Input: part model. Units: mm. Frame: model coordinates. Face numbers are marked on the shaded views. A direction names the side the tool comes from. Give positions to 0.01 mm unless a question says otherwise; leave off trailing zeros. Loops run counter-clockwise (first coordinate to the right, second up) from the corner with the lowest first, then second, coordinate; pieces in that order, holes last. Notation, with made-up numbers: (9.5, 78.25) - (66.5, 78.25) arc R32 cw to (66.5, 112.25) - close; hole circle Ø3 at (-13, 9.25). An arc over 180 degrees is marked (long way). Answer as a JSON object with one key per item and string values.
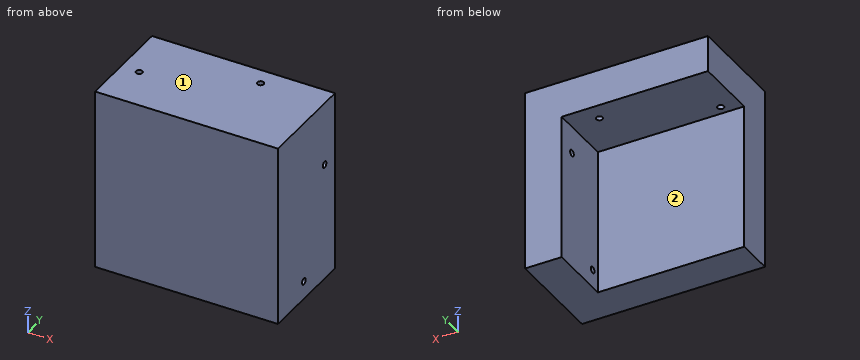
Autodesk Inventor part; units mm, degrees
ref_plane "YZ Plane" through (0, 0, 0) normal (1, 0, 0) x (0, 1, 0)
ref_plane "XZ Plane" through (0, 0, 0) normal (0, 1, 0) x (-1, 0, 0)
ref_plane "XY Plane" through (0, 0, 0) normal (0, 0, 1) x (1, 0, 0)
sketch "Boceto2" plane through (0, 0, 0) normal (0, 1, 0) x (-1, 0, 0)
  line L0 (7.5, 100) -> (-7.5, 100)
  line L1 (-7.5, 100) -> (-7.5, -100)
  line L2 (-7.5, -100) -> (7.5, -100)
  line L3 (7.5, -100) -> (7.5, 100)
  line L4 (7.5, 100) -> (-7.5, -100) construction
  line L5 (-7.5, 100) -> (7.5, -100) construction
  point P0 (0, 0)
  dimension "d7" = 15
  dimension "d8" = 200
extrude "Extrusión1" add sketch "Boceto2" along normal blind 10
sketch "Boceto3" plane through (0, 10, 0) normal (0, 1, 0) x (1, 0, 0)
  circle A0 centre (3.25, 58.25) radius 1.75
  line L0 (5, 50) -> (-5, 50)
  line L1 (-5, 50) -> (-5, 60)
  line L2 (-5, 60) -> (5, 60)
  line L3 (5, 60) -> (5, 50)
  line L4 (5, 50) -> (-5, 60) construction
  line L5 (-5, 50) -> (5, 60) construction
  circle A1 centre (-3.25, 51.75) radius 1.75
  line L6 (7.5, 100) -> (-7.5, 100)
  line L7 (-7.5, 0) -> (3.408, 0)
  line L8 (5, -60) -> (5, -50)
  line L9 (-5, -60) -> (5, -60)
  line L10 (5, -50) -> (-5, -50)
  line L11 (-5, -50) -> (-5, -60)
  line L12 (-5, -50) -> (5, -60) construction
  circle A2 centre (-3.25, -51.75) radius 1.75
  line L13 (5, -50) -> (-5, -60) construction
  circle A3 centre (3.25, -58.25) radius 1.75
  line L14 (-7.5, -100) -> (7.5, -100)
  point P0 (0, 0)
  point P1 (-5, 55)
  point P2 (0, 100)
  point P3 (-5, -55)
  dimension "d11" = 3.5
  dimension "d12" = 1.75
  dimension "d13" = 1.75
  dimension "d14" = 1.75
  dimension "d15" = 1.75
  dimension "d16" = 10
  dimension "d17" = 10
  dimension "d19" = 40
  dimension "d81" = 40
hole "Agujero1" at (3.25, 10, 58.25) at (-3.25, 10, 51.75) at (3.25, 10, -58.25) at (-3.25, 10, -51.75) direction (0, -1, 0) diameter 3.5 end through all
sketch "Boceto4" plane through (0, 10, 0) normal (0, 1, 0) x (1, 0, 0)
  line L0 (-7.5, 100) -> (-7.5, -100)
  line L1 (-7.5, -100) -> (7.5, -100)
  line L2 (7.5, -100) -> (7.5, -80)
  line L3 (7.5, -80) -> (-7.5, -80)
  line L4 (-7.5, -80) -> (-7.5, -100)
  line L5 (-7.5, 0) -> (1.0116, 0)
  line L6 (-7.5, -100) -> (-7.5, 100)
  line L7 (-7.5, 100) -> (7.5, 100)
  line L8 (7.5, 100) -> (7.5, 80)
  line L9 (7.5, 80) -> (-7.5, 80)
  line L10 (-7.5, 80) -> (-7.5, 100)
  point P0 (0, 0)
  point P1 (-7.5, -80)
  point P2 (-7.5, 80)
  dimension "d27" = 15
  dimension "d28" = 20
extrude "Extrusión2" add sketch "Boceto4" along normal blind 80
sketch "Boceto5" plane through (0, 90, 0) normal (0, 1, 0) x (1, 0, 0)
  line L0 (-7.5, -100) -> (7.5, -100)
  line L1 (-7.5, -100) -> (49.5, -100)
  line L2 (49.5, -100) -> (49.5, 100)
  line L3 (49.5, 100) -> (-7.5, 100)
  line L4 (-7.5, 100) -> (-7.5, -100)
  line L5 (49.5, -100) -> (-150.5, -100)
  line L6 (-150.5, -100) -> (-150.5, 100)
  line L7 (-150.5, 100) -> (49.5, 100)
  line L8 (49.5, 100) -> (49.5, -100)
  point P0 (0, 0)
  point P1 (-7.5, 100)
  dimension "d31" = 57
  dimension "d32" = 200
  dimension "d75" = 200
extrude "Extrusión3" add sketch "Boceto5" along normal blind 110
sketch "Boceto6" plane through (0, 200, 0) normal (0, 1, 0) x (1, 0, 0)
  line L0 (49.5, 100) -> (7.5, 100)
  line L1 (49.5, 100) -> (29.5, 100)
  line L2 (29.5, 100) -> (29.5, 80)
  line L3 (7.5, -100) -> (49.5, -100)
  line L4 (28.5, -100) -> (28.5, -80)
  line L5 (-150.5, 100) -> (-150.5, -100)
  line L6 (29.5, 80) -> (-150.5, 80)
  line L7 (-150.5, 80) -> (-150.5, -80)
  line L8 (-150.5, -80) -> (29.5, -80)
  line L9 (29.5, -80) -> (29.5, 80)
  line L10 (-150.5, -100) -> (49.5, -100)
  point P0 (7.5, 80)
  point P1 (-50.5, -100)
  dimension "d36" = 20
  dimension "d37" = 20
  dimension "d38" = 20
  dimension "d77" = 20
extrude "Extrusión4" cut sketch "Boceto6" against normal blind 90 contours L8 L5 L6 L9
sketch "Boceto7" plane through (-150.5, 90, -100) normal (-1, 0, 0) x (0, 0, 1)
  line L0 (0, 110) -> (20, 110)
  line L1 (20, 110) -> (10, 110)
  line L2 (10, 110) -> (10, 20)
  line L3 (10, 20) -> (20, 20)
  line L4 (20, 20) -> (20, 110)
  line L5 (180, 110) -> (180, 20)
  line L6 (180, 110) -> (190, 110)
  line L7 (190, 110) -> (190, 20)
  line L8 (190, 20) -> (180, 20)
  line L9 (180, 20) -> (180, 110)
  line L10 (200, 0) -> (200, 110)
  line L11 (0, 0) -> (0, 110)
  line L12 (0, 110) -> (10, 110)
  line L13 (10, 110) -> (10, 20)
  line L14 (10, 20) -> (0, 20)
  line L15 (0, 20) -> (0, 110)
  line L16 (200, 110) -> (0, 110)
  line L17 (200, 110) -> (190, 110)
  line L18 (190, 110) -> (190, 20)
  line L19 (190, 20) -> (200, 20)
  line L20 (200, 20) -> (200, 110)
  point P0 (100, -90)
  dimension "d63" = 10
  dimension "d65" = 10
  dimension "d76" = 10
extrude "Extrusión5" cut sketch "Boceto7" against normal blind 30 contours L6 L7 L8 L5 | L0 L4 L3 L2
sketch "Boceto8" plane through (-7.5, 0, 100) normal (0, 0, 1) x (1, 0, 0)
  line L0 (-113, 110) -> (-113, 200)
  line L1 (-113, 200) -> (-113, 110)
  circle A0 centre (-124.75, 183.25) radius 1.75
  line L2 (-123, 175) -> (-133, 175)
  line L3 (-133, 175) -> (-133, 185)
  line L4 (-133, 185) -> (-123, 185)
  line L5 (-123, 185) -> (-123, 175)
  line L6 (-123, 175) -> (-133, 185) construction
  line L7 (-133, 175) -> (-123, 185) construction
  circle A1 centre (-131.25, 176.75) radius 1.75
  line L8 (-143, 200) -> (57, 200)
  line L9 (-143, 90) -> (-143, 200)
  line L10 (-113, 155) -> (-128, 155)
  line L11 (-123, 125) -> (-123, 135)
  line L12 (-133, 125) -> (-123, 125)
  line L13 (-123, 135) -> (-133, 125) construction
  line L14 (-123, 135) -> (-133, 135)
  line L15 (-133, 135) -> (-123, 125) construction
  circle A2 centre (-131.25, 133.25) radius 1.75
  line L16 (-133, 135) -> (-133, 125)
  circle A3 centre (-124.75, 126.75) radius 1.75
  line L17 (-143, 110) -> (-113, 110)
  point P0 (7.5, 0)
  point P1 (-133, 180)
  point P2 (-123, 180)
  point P3 (-133, 130)
  point P4 (-123, 130)
  dimension "d45" = 3.5
  dimension "d46" = 1.75
  dimension "d47" = 1.75
  dimension "d48" = 1.75
  dimension "d49" = 1.75
  dimension "d50" = 10
  dimension "d51" = 10
  dimension "d52" = 15
  dimension "d53" = 10
  dimension "d54" = 10
  dimension "d55" = 15
hole "Agujero2" at (-132.25, 183.25, 100) at (-138.75, 176.75, 100) at (-138.75, 133.25, 100) at (-132.25, 126.75, 100) direction (0, 0, -1) diameter 3.5 end through all
ref_plane "Plano de trabajo1" through (-150.5, 90, 100) normal (0, -1, 0) x (1, 0, 0)
split "Dividir1" plane through (-150.5, 90, 100) removes the side toward (0, -1, 0)
ref_plane "Plano de trabajo2" through (49.5, 90, 0) normal (0, 0, -1) x (-1, 0, 0)
ref_plane "Plano de trabajo3" through (-50.5, 90, 100) normal (1, 0, 0) x (0, 0, -1)
ref_plane "Plano de trabajo4" through (0, 145, 0) normal (0, 1, 0) x (1, 0, 0)
sketch "Boceto9" plane through (-150.5, 90, 100) normal (0, 0, 1) x (1, 0, 0)
  line L0 (85.0357, 30) -> (115.0357, 30)
  circle A0 centre (110.0357, 25) radius 1.75
  line L1 (90.0357, 25) -> (110.0357, 25)
  line L2 (115.0357, 30) -> (115.0357, 20)
  circle A1 centre (90.0357, 25) radius 1.75
  line L3 (85.0357, 20) -> (115.0357, 30) construction
  line L4 (85.0357, 30) -> (115.0357, 20) construction
  line L5 (85.0357, 20) -> (85.0357, 30)
  line L6 (115.0357, 20) -> (85.0357, 20)
  line L7 (200, 0) -> (200, 110)
  line L8 (200, 55) -> (88.2857, 55)
  circle A2 centre (90.0357, 85) radius 1.75
  line L9 (85.0357, 80) -> (115.0357, 80)
  line L10 (85.0357, 80) -> (115.0357, 90) construction
  line L11 (85.0357, 90) -> (85.0357, 80)
  line L12 (115.0357, 90) -> (85.0357, 90)
  line L13 (85.0357, 90) -> (115.0357, 80) construction
  circle A3 centre (110.0357, 85) radius 1.75
  line L14 (90.0357, 85) -> (110.0357, 85)
  line L15 (115.0357, 80) -> (115.0357, 90)
  line L16 (100.0357, 55) -> (185.099, 55) construction
  line L17 (160, 70) -> (160, 40)
  circle A4 centre (165, 45) radius 1.75
  line L18 (170, 40) -> (170, 70)
  line L19 (170, 70) -> (160, 40) construction
  line L20 (160, 40) -> (170, 40)
  line L21 (160, 70) -> (170, 40) construction
  circle A5 centre (165, 65) radius 1.75
  line L22 (165, 65) -> (165, 45)
  line L23 (170, 70) -> (160, 70)
  circle A6 centre (55, 65) radius 1.75
  line L24 (60, 70) -> (60, 40)
  line L25 (60, 40) -> (50, 40)
  circle A7 centre (55, 45) radius 1.75
  line L26 (55, 65) -> (55, 45)
  line L27 (60, 70) -> (50, 40) construction
  line L28 (50, 40) -> (50, 70)
  line L29 (50, 70) -> (60, 40) construction
  line L30 (50, 70) -> (60, 70)
  line L31 (30, 110) -> (30, 20)
  point P0 (150.5, -90)
  point P1 (100.0357, 34.7141)
  point P2 (100.0357, 34.7141)
  point P3 (85.0357, 36.6749)
  point P4 (115.0357, 25)
  point P5 (115.0357, 85)
  point P6 (189.1833, 40)
  point P7 (165, 70)
  point P8 (70.0357, 40)
  point P9 (55, 70)
  dimension "d89" = 10
  dimension "d90" = 30
  dimension "d91" = 5
  dimension "d92" = 5
  dimension "d93" = 5
  dimension "d94" = 5
  dimension "d95" = 30
  dimension "d96" = 5
  dimension "d97" = 5
  dimension "d98" = 3.5
  dimension "d99" = 5
  dimension "d100" = 5
  dimension "d101" = 5
  dimension "d102" = 5
  dimension "d103" = 5
  dimension "d104" = 20
hole "Agujero3" at (-60.4643, 175, 100) at (-40.4643, 175, 100) at (14.5, 155, 100) at (-95.5, 155, 100) at (-95.5, 135, 100) at (-60.4643, 115, 100) at (-40.4643, 115, 100) at (14.5, 135, 100) direction (0, 0, -1) diameter 3.5 end through all
sketch "Boceto10" plane through (49.5, 90, 100) normal (1, 0, 0) x (0, 0, -1)
  line L0 (85.0357, 30) -> (115.0357, 30)
  circle A0 centre (110.0357, 25) radius 1.75
  line L1 (90.0357, 25) -> (110.0357, 25)
  line L2 (115.0357, 30) -> (115.0357, 20)
  circle A1 centre (90.0357, 25) radius 1.75
  line L3 (85.0357, 30) -> (115.0357, 20) construction
  line L4 (85.0357, 20) -> (85.0357, 30)
  line L5 (115.0357, 20) -> (85.0357, 20)
  line L6 (85.0357, 20) -> (115.0357, 30) construction
  line L7 (160, 70) -> (160, 40)
  circle A2 centre (165, 45) radius 1.75
  line L8 (160, 40) -> (170, 40)
  line L9 (165, 65) -> (165, 45)
  circle A3 centre (165, 65) radius 1.75
  line L10 (170, 70) -> (160, 40) construction
  line L11 (170, 70) -> (160, 70)
  line L12 (160, 70) -> (170, 40) construction
  line L13 (170, 40) -> (170, 70)
  line L14 (40, 70) -> (40, 40)
  line L15 (35, 65) -> (35, 45)
  circle A4 centre (35, 65) radius 1.75
  line L16 (40, 40) -> (30, 40)
  line L17 (40, 70) -> (30, 40) construction
  line L18 (30, 70) -> (40, 40) construction
  line L19 (30, 70) -> (40, 70)
  line L20 (30, 40) -> (30, 70)
  circle A5 centre (35, 45) radius 1.75
  circle A6 centre (90.0357, 85) radius 1.75
  line L21 (85.0357, 80) -> (115.0357, 80)
  line L22 (115.0357, 80) -> (115.0357, 90)
  circle A7 centre (110.0357, 85) radius 1.75
  line L23 (90.0357, 85) -> (110.0357, 85)
  line L24 (85.0357, 80) -> (115.0357, 90) construction
  line L25 (85.0357, 90) -> (85.0357, 80)
  line L26 (115.0357, 90) -> (85.0357, 90)
  line L27 (85.0357, 90) -> (115.0357, 80) construction
  line L28 (0, 0) -> (0, 110)
  line L29 (200, 0) -> (200, 110)
  point P0 (100, -90)
  point P1 (100.0357, 34.7141)
  point P2 (100.0357, 34.7141)
  point P3 (85.0357, 36.6749)
  point P4 (115.0357, 25)
  point P5 (88.2857, 55)
  point P6 (189.1833, 40)
  point P7 (165, 70)
  point P8 (70.0357, 40)
  point P9 (35, 70)
  point P10 (115.0357, 85)
  point P11 (100.0357, 55)
  dimension "d112" = 10
  dimension "d113" = 30
  dimension "d114" = 5
  dimension "d115" = 5
  dimension "d116" = 5
  dimension "d117" = 5
  dimension "d118" = 5
  dimension "d119" = 5
  dimension "d120" = 3.5
  dimension "d121" = 5
  dimension "d122" = 5
  dimension "d123" = 5
  dimension "d124" = 5
  dimension "d125" = 5
  dimension "d126" = 30
  dimension "d127" = 30
hole "Agujero4" at (49.5, 175, 9.9643) at (49.5, 175, -10.0357) at (49.5, 155, 65) at (49.5, 135, 65) at (49.5, 115, 9.9643) at (49.5, 115, -10.0357) at (49.5, 135, -65) at (49.5, 155, -65) direction (-1, 0, 0) diameter 3.5 end through all
split "Dividir2" plane through (-50.5, 90, 100) removes the side toward (-1, 0, 0)
split "Dividir3" plane through (0, 145, 0) removes the side toward (0, 1, 0)
split "Dividir4" plane through (49.5, 90, 0) removes the side toward (0, 0, -1)
properties part number "container_front_head_2"
Item 1: Cut plane B-B (y = 135). Return loops of the section in (x, z).
Geometry check:
{"outline": "(-50.5, 80) - (12.75, 80) - (12.75, 100) - (-50.5, 100) - close; (16.25, 80) - (29.5, 80) - (29.5, 66.75) - (49.5, 66.75) - (49.5, 100) - (16.25, 100) - close; (29.5, 0) - (49.5, 0) - (49.5, 63.25) - (29.5, 63.25) - close"}
Item 2: Access query for the marked faces 1 and 2. Directions: +Z, -Z, +X, -X, +Y, -Y. A direction counts if a zero-diameter tool reaches every point of the face in a straight line with its end or side. Return the directions, or none.
Geometry check:
{"face 1": "+Z, +X, -X, +Y, -Y", "face 2": "-Z, -X, +Y"}
Item 3: Cut plane A-A (z = 65). Return loops of the section in (x, y).
Geometry check:
{"outline": "(-50.5, 90) - (49.5, 90) - (49.5, 133.25) - (29.5, 133.25) - (29.5, 110) - (-50.5, 110) - close; (29.5, 136.75) - (49.5, 136.75) - (49.5, 145) - (29.5, 145) - close"}
Item 4: Contact query for flat-ended pins moving along their axis: P1, Ø3, axis at x = -4.5, z = 60.5, coming from the +Y side; P2, Ø17.5, axis at x = 0, y = 128, coming from the -Z side; P3, Ø4.5, axis at y = 115, z = 9.96, coming from the -X side. Output: stop coordinate, or through.
Geometry check:
{"P1": "stops at y = 110", "P2": "stops at z = 80", "P3": "stops at x = 29.5"}
Item 5: Material intervals for line 1 (X direction, y = 115, z = 90.5); line 2 (Y direction, x = 42, z = 65); line 3 (Y direction, x = 26.5, z = 50), sorted ascending. Write a range as [from, to].
Geometry check:
{"line 1": "x = [-50.5, -42.21], [-38.71, 49.5]", "line 2": "y = [90, 133.25], [136.75, 145]", "line 3": "y = [90, 110]"}
Item 6: Cut plane D-D (z = 17). Return loops of the section in (x, y), then the cut area to 3 significant figures.
Geometry check:
{"outline": "(-50.5, 90) - (49.5, 90) - (49.5, 145) - (29.5, 145) - (29.5, 110) - (-50.5, 110) - close", "area": "2,700 mm2"}
Item 7: Cut plane C-C (x = 8). Return loops of the section in (y, z).
Geometry check:
{"outline": "(90, 0) - (110, 0) - (110, 80) - (145, 80) - (145, 100) - (90, 100) - close"}
